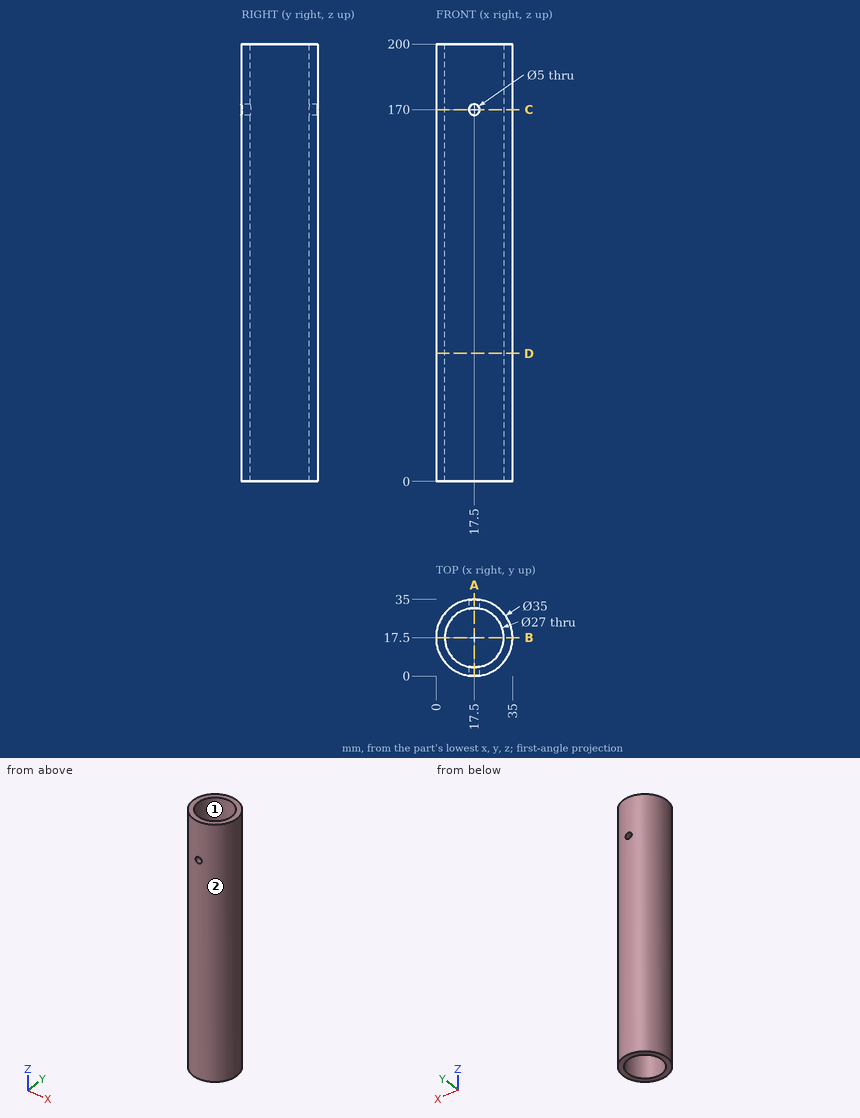
Geometry check sheet. Reference: drawing and pictorial views, mm from the part's lowest x, y, z. Give positions to 0.01 mm unless a question says otherwise; leave off trailing zeros. Loops run counter-clockwise (first coordinate to the right, second up) from the corner with the lowest first, then second, coordinate; pieces in that order, holes last. Notation, with made-up numbers: M -28,-2.5 L -6,-2.5 A15 cw -6,20.5 Z; hole C 10,-10 d6. An arc over 180 degrees is marked long. Use a Markdown table: item, result. Add a question column.
Q1. Sectioned sample at D-D, the plane z = 58.5. Record the cut outline in (x, y), then the cut area to 3 significant figures.
Q2. Sectioned sample at B-B, the plane y = 17.5. Record the cut outline in (x, z), then the cut area to 3 significant figures.
Q3. Sectioned sample at A-A, the plane x = 17.5. Record the cut outline in (y, z).
Q4. Sectioned sample at C-C, the plane z = 170. Record the cut outline in (x, y).
Q5. Scan lines: line 1 along Z through (x, y) = (17.5, 2.3); line 2 along Y through (x, z) = (17.5, 158); line 3 along X through (y, z) = (5, 183.5). Record each from-to range of solid material in increasing order. Write a range as [from, to].
Q6. Mould release check, pull along Y, two halves, no side actions. Record for the marked faces 1 and 2: pulls with the +Y half, pulls with the -Y half, needs draft (parallel to the pull), parting line crosses it, or undercut.
Q7. Go/stop test with flat-tipped pins: pin 1 (1.5 mm diameter, centred on x = 22.5, z = 131.5, fed in from +Y); pin 2 (6 mm diameter, centred on x = 11, z = 97, fed in from -Y); pin 3 (12 mm diameter, centred on x = 27, z = 61, fed in from +Y). Record where each tip stops, or that it passes through.
Verdict:
| question | item | result |
|---|---|---|
| 1 | outline | C 17.5,17.5 d35; hole C 17.5,17.5 d27 |
| 1 | area | 390 mm^2 |
| 2 | outline | M 0,0 L 4,0 L 4,200 L 0,200 Z; M 31,0 L 35,0 L 35,200 L 31,200 Z |
| 2 | area | 1,600 mm^2 |
| 3 | outline | M 0,0 L 4,0 L 4,167.5 L 0,167.5 Z; M 0,172.5 L 4,172.5 L 4,200 L 0,200 Z; M 31,0 L 35,0 L 35,167.5 L 31,167.5 Z; M 31,172.5 L 35,172.5 L 35,200 L 31,200 Z |
| 4 | outline | M 15,0.18 L 15,4.23 A13.5 cw 15,30.77 L 15,34.82 A17.5 ccw Z; M 20,0.18 A17.5 ccw 20,34.82 L 20,30.77 A13.5 cw 20,4.23 Z |
| 5 | line 1 | [0, 167.5], [172.5, 200] |
| 5 | line 2 | [0, 4], [31, 35] |
| 5 | line 3 | [5.25, 12.4], [22.6, 29.75] |
| 6 | face 1 | undercut |
| 6 | face 2 | parting line crosses it |
| 7 | pin 1 | y = 34.48 |
| 7 | pin 2 | y = 0.35 |
| 7 | pin 3 | y = 34.65 |
